Input: part model. Units: mm. Frame: model coordinates. Face numbers are marked on the shaded views. A direction names the side the tool comes from. Give positions to 0.01 mm unless a question says otherwise; leave off trailing zeros. Loops run counter-clockwise (first coordinate to the right, second up) from the corner with the lowest first, then second, coordinate; pieces in that order, holes last.
from build123d import *

# Parameters (mm, degrees)
CROQUIS1_W                       = 100
CROQUIS1_H                       = 75
SALIENTE_EXTRUIR1_DEPTH          = 40
CROQUIS2_W                       = 90
CROQUIS2_H                       = 65
CORTAR_EXTRUIR1_DEPTH            = 105.472453923
CROQUIS3_W                       = 90
CROQUIS3_H                       = 65
SALIENTE_EXTRUIR2_DEPTH          = 5
TALADRO_DE_MARGEN_PARA_M31_D     = 3.4
TALADRO_DE_MARGEN_PARA_M31_DEPTH = 20
TALADRO_DE_MARGEN_PARA_M31_TIP   = 1.021463052


with BuildPart() as part:
    # Croquis1 → Saliente-Extruir1 (new body)
    with BuildSketch(Plane(origin=(0, 0, 0), x_dir=(1, 0, 0), z_dir=(0, 1, 0))):
        with Locations((25.018270402, -23.21863581)):
            Rectangle(CROQUIS1_W, CROQUIS1_H)
    extrude(amount=SALIENTE_EXTRUIR1_DEPTH)

    # Croquis2 → Cortar-Extruir1 (cut, through all)
    with BuildSketch(Plane(origin=(0, 0, 0), x_dir=(1, 0, 0), z_dir=(0, 1, 0))):
        with Locations((25.018270402, -23.21863581)):
            Rectangle(CROQUIS2_W, CROQUIS2_H)
    extrude(amount=CORTAR_EXTRUIR1_DEPTH, mode=Mode.SUBTRACT)

    # Croquis3 → Saliente-Extruir2 (add)
    with BuildSketch(Plane(origin=(0, 0, 0), x_dir=(1, 0, 0), z_dir=(0, 1, 0))):
        with Locations((25.018270402, -23.21863581)):
            Rectangle(CROQUIS3_W, CROQUIS3_H)
    extrude(amount=SALIENTE_EXTRUIR2_DEPTH)

    # Taladro de margen para M31
    with Locations(Plane(origin=(-22.481719301, 40, -11.781363893), x_dir=(0, 0, 1), z_dir=(0, 1, 0))):
        with Locations((0, 0), (-2.33e-07, 94.999989703), (69.999999703, 94.999989703), (69.999999703, 1.038e-06)):
            Hole(TALADRO_DE_MARGEN_PARA_M31_D / 2, depth=TALADRO_DE_MARGEN_PARA_M31_DEPTH)
            with Locations((0, 0, -(TALADRO_DE_MARGEN_PARA_M31_DEPTH + TALADRO_DE_MARGEN_PARA_M31_TIP / 2))):  # 118° drill point
                Cone(0, TALADRO_DE_MARGEN_PARA_M31_D / 2, TALADRO_DE_MARGEN_PARA_M31_TIP, mode=Mode.SUBTRACT)


solid = part.part
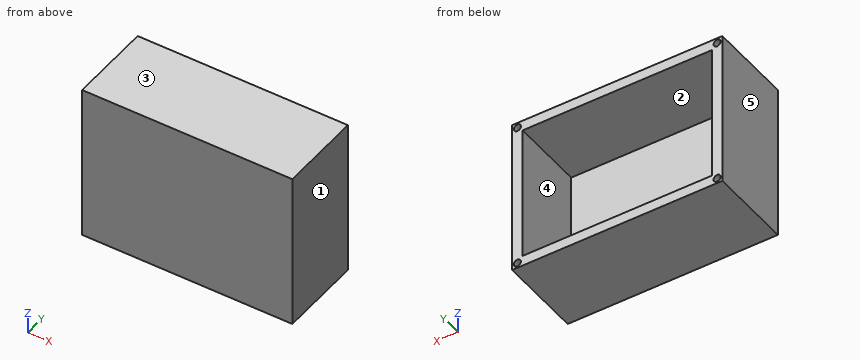
(1) Mould query, pull axis X, two halves, no side actions, for the marked faces 1, 2 and 3. Classes: +X half, -X half, draft (parallel to the pull), parting line (faces both ways), or undercut.
Values follow:
face 1: +X half
face 2: undercut
face 3: draft
(2) Cut plane D-D (y = 37). Return the cut outline in (x, z).
Values follow:
outline: (-24.98, -14.28) - (75.02, -14.28) - (75.02, 60.72) - (-24.98, 60.72) - close; hole circle Ø3.4 at (-22.48, -11.78); hole circle Ø3.4 at (-22.48, 58.22); hole (-19.98, -9.28) - (70.02, -9.28) - (70.02, 55.72) - (-19.98, 55.72) - close; hole circle Ø3.4 at (72.52, -11.78); hole circle Ø3.4 at (72.52, 58.22)
(3) Cut plane A-A (z = 18). Return the cut outline in (x, y).
Values follow:
outline: (-24.98, 0) - (75.02, 0) - (75.02, 40) - (70.02, 40) - (70.02, 5) - (-19.98, 5) - (-19.98, 40) - (-24.98, 40) - close
(4) Cut plane B-B (y = 12.5). Return the cut outline in (x, z), and give its area (3 significant figures).
Values follow:
outline: (-24.98, -14.28) - (75.02, -14.28) - (75.02, 60.72) - (-24.98, 60.72) - close; hole (-19.98, -9.28) - (70.02, -9.28) - (70.02, 55.72) - (-19.98, 55.72) - close
area: 1,650 mm2
(5) Ray query, probe 1 along X at (y, z) = (38.5, 11); probe 2 along Z at (x, y) = (16.5, 26.5); probe 3 along Y at (x, z) = (23, 24). Return the intervals inside material, ascending.
Values follow:
probe 1: x = -24.98 to -19.98, 70.02 to 75.02
probe 2: z = -14.28 to -9.28, 55.72 to 60.72
probe 3: y = 0 to 5
(6) Reachability of the marked faces 4 and 5 from +Z, -Z, +X, -X, +Y, -Y: full face, straight path, thin tool, end or side. Return the list, or none.
Values follow:
face 4: +Y
face 5: +Z, -Z, -X, +Y, -Y
(7) Cut plane C-C (x = 40.5). Return the cut outline in (y, z), and give its area (3 significant figures).
Values follow:
outline: (0, -14.28) - (40, -14.28) - (40, -9.28) - (5, -9.28) - (5, 55.72) - (40, 55.72) - (40, 60.72) - (0, 60.72) - close
area: 725 mm2
(8) Pin query (flat end, axial travel): pin 1 Ø5.5 at (x, z) = (72.52, 58.22) entering from +Y; pin 2 Ø3 at (x, z) = (72.52, -11.78) entering from +Y; pin 3 Ø2.5 at (x, z) = (-22.48, 58.22) entering from +Y; pin 4 Ø12 at (x, z) = (36.5, 32) entering from +Y. Return the tip coordinate at first contact, or that it passes through.
Values follow:
pin 1: stops at y = 40
pin 2: stops at y = 19.88
pin 3: stops at y = 19.73
pin 4: stops at y = 5
